```python
from build123d import *

# Parameters (mm, degrees)
SKETCH1_R           = 1.25
BOSS_EXTRUDE1_DEPTH = 10


with BuildPart() as part:
    # Sketch1 → Boss-Extrude1 (new body)
    # profile 1 of 2: a face of its own
    with BuildSketch(Plane(origin=(0, 0, 0), x_dir=(1, 0, 0), z_dir=(0, 1, 0))):
        Polygon((6, 55), (3, 55), (0, 55), (0, 0), (6, 0), (6, 6), align=None)
        with BuildLine():
            ThreePointArc((4.25, 40), (2.116116524, 39.116116524), (3, 41.25))
            ThreePointArc((3, 41.25), (3.883883476, 40.883883476), (4.25, 40))
        make_face(mode=Mode.SUBTRACT)
    # profile 2 of 2: a face of its own
    with BuildSketch(Plane(origin=(0, 0, 0), x_dir=(1, 0, 0), z_dir=(0, 1, 0))):
        Polygon((30.028010211, 6), (6, 6), (6, 0), (30.028010211, 0), (30.028010211, 3), align=None)
        with Locations(Location((25.028010211, 3, 0), (0, 0, 270))):
            Circle(SKETCH1_R, mode=Mode.SUBTRACT)
    extrude(amount=BOSS_EXTRUDE1_DEPTH)


solid = part.part
```
CAD build for the part. Positions are in the model's coordinates, mm. A direction names the side the tool comes from. Round coordinates to 2 decimals unless told otherwise and drop trailing zeros. Loops run counter-clockwise (first coordinate to the right, second up) from the corner with the lowest first, then second, coordinate; pieces in that order, holes last. Notation, with made-up numbers: (-22.75, 33) - (34.25, 33) arc R21 cw to (34.25, 43) - close; hole circle Ø8 at (88.25, -28.5). An arc over 180 degrees is marked (long way). Return JSON: item names as keys, results as strings. Group by question number.
Q1. Two-plate mould, pull along Z, no slides. Class faces 3 (the face through (15, 5, 0)), 4 (the face through (23.808, 4.93, -3.271)), 5 (the face through (18, 5, -6)): +Z half, -Z half, draft (parallel to the pull), parting line (faces both ways), or undercut.
Q2. Tool access for faces 1 (the face through (6, 5, -30)), 2 (the face through (5, 10, -22)): list every direction of +Z, -Z, +X, -X, +Y, -Y with a clear straight run to the whole face (end or side of a thin tool).
Q3. Flat gauge pin, fed straight in: pin 1 Ø1 at (x, y) = (12.5, 7) entering from -Z. Where does the tip first touch, or does it go through?
Q4. Drill centre lines: line 1 along X through (y, z) = (6, -3); line 2 along Z through (x, y) = (3, 7.25); line 3 along X through (y, z) = (2.75, -40). Where is each one in solid material? Low to high. Write a range as [from, to].
Q5. Band-saw the part on A-A on z = -3. Give the cut face in (x, y).
Q6. Band-saw the part on C-C on x = 15. Give the cut face in (y, z).
Q7. Band-saw the part on B-B on z = -21.5. Give the cut face in (x, y).
Solutions:
{
 "1": {"face 3": "+Z half", "face 4": "undercut", "face 5": "-Z half"},
 "2": {"face 1": "-Z, +X, +Y, -Y", "face 2": "+Z, -Z, +X, -X, +Y"},
 "3": {"pin 1": "stops at z = -6"},
 "4": {"line 1": "x = [0, 23.78], [26.28, 30.03]", "line 2": "z = [-55, -41.25], [-38.75, 0]", "line 3": "x = [0, 1.75], [4.25, 6]"},
 "5": {"outline": "(0, 0) - (23.78, 0) - (23.78, 10) - (0, 10) - close; (26.28, 0) - (30.03, 0) - (30.03, 10) - (26.28, 10) - close"},
 "6": {"outline": "(0, -6) - (10, -6) - (10, 0) - (0, 0) - close"},
 "7": {"outline": "(0, 0) - (6, 0) - (6, 10) - (0, 10) - close"}
}
